Can you work these out from the model? Positions are in its coordinate system, mm. A direction names the side the tool comes from. Coordinates: 2 decimals unless noted, no trailing zeros. Order: outer loops, then holes, each group sorted by start corner. A loop starts at its lowest first (then second) coordinate and runs counter-clockwise, first axis right, second up. Notation, with made-up numbers: (39, 73) -> (44, 73) arc R22 ccw to (44, 96) -> close; hole circle Ø3 at (44, -30). An arc over 180 degrees is marked (long way). Write item = value, one per line.
```python
from build123d import *

# Parameters (mm, degrees)
SKETCH_R          = 1.5
PAD_DEPTH         = 8
SKETCH001_W       = 18.9
SKETCH001_H       = 25.2
POCKET_DEPTH      = 0.8
SKETCH002_W       = 15
SKETCH002_H       = 2.5
SKETCH002_W_2     = 10.4
POCKET001_DEPTH   = 3
SKETCH003_W       = 6
SKETCH003_H       = 30
PAD001_DEPTH      = 9
SKETCH004_W       = 19.2
SKETCH004_H       = 1
POCKET002_DEPTH   = 2
POCKET003_DEPTH   = 3
PAD002_DEPTH      = 3
PAD002_DEPTH_BACK = 3
PAD003_DEPTH      = 1
CHAMFER_SIZE      = 0.95


with BuildPart() as part:
    # Sketch → Pad (new body)
    with BuildSketch(Plane.XY):
        Polygon((-20.1, 15), (11.9, 15), (30, 3.75), (30, -3.75), (11.9, -15), (-20.1, -15), align=None)
        with Locations((-6.25, 0)):
            Circle(SKETCH_R, mode=Mode.SUBTRACT)
    extrude(amount=-PAD_DEPTH)

    # Sketch001 → Pocket (cut)
    with BuildSketch(Plane.XY):
        Rectangle(SKETCH001_W, SKETCH001_H)
    extrude(amount=-POCKET_DEPTH, mode=Mode.SUBTRACT)

    # Sketch002 (on Face33 of Pad003) → Pocket001 (cut)
    with BuildSketch(Plane.XY.offset(-0.8)):
        with Locations((-0.534042, 8.083783)):
            Rectangle(SKETCH002_W, SKETCH002_H)
        with Locations((2.090713, -8.153236)):
            Rectangle(SKETCH002_W_2, SKETCH002_H)
    extrude(amount=-POCKET001_DEPTH, mode=Mode.SUBTRACT)

    # Sketch003 (on Face4 of Pocket001) → Pad001 (join)
    with BuildSketch(Plane.XY):
        with Locations((-17.1, 0)):
            Rectangle(SKETCH003_W, SKETCH003_H)
    extrude(amount=PAD001_DEPTH)

    # Sketch004 (on Face10 of Pad001) → Pocket002 (cut)
    with BuildSketch(Plane.YZ.offset(-14.1)):
        with Locations((0, 5.64)):
            Rectangle(SKETCH004_W, SKETCH004_H)
    extrude(amount=-POCKET002_DEPTH, mode=Mode.SUBTRACT)

    # Sketch005 → Pocket003 (cut)
    with BuildSketch(Plane(origin=(0, 0, -8), x_dir=(1, 0, 0), z_dir=(0, 0, -1))):
        Polygon((-4.633419, 2.8), (-7.866581, 2.8), (-9.483162, 0), (-7.866581, -2.8), (-4.633419, -2.8), (-3.016838, 0), align=None)
    extrude(amount=-POCKET003_DEPTH, mode=Mode.SUBTRACT)

    # Sketch006 → Pad002 (join, two sides)
    with BuildSketch(Plane.XZ) as pad002_sk:
        Polygon((13.9, 0), (20.9, 5.25), (26.9, 5.25), (26.9, 0), align=None)
    extrude(amount=PAD002_DEPTH)
    extrude(pad002_sk.sketch, amount=-PAD002_DEPTH_BACK)

    # Sketch007 (on Face32 of Pad002) → Pad003 (join)
    with BuildSketch(Plane.XY.offset(5.25)):
        with BuildLine():
            ThreePointArc((24, -1.925), (25.925, 0), (24, 1.925))
            Line((24, 1.925), (23, 1.925))
            Line((23, 1.925), (23, -1.925))
            Line((23, -1.925), (24, -1.925))
        make_face()
    extrude(amount=PAD003_DEPTH)

    # Chamfer
    chamfer_edges = [part.edges().sort_by_distance(p)[0] for p in [
        (23, 0, 6.25),
        (23, -1.925, 5.75),
        (23, 1.925, 5.75),
    ]]
    chamfer(chamfer_edges, length=CHAMFER_SIZE)


solid = part.part
```
Item 1: I want a section at A-A, the plane x = -6.25. Please give me the cut outline in (y, z).
A:
outline = (-15, -8) -> (-2.8, -8) -> (-2.8, -5) -> (-1.5, -5) -> (-1.5, -0.8) -> (-12.6, -0.8) -> (-12.6, 0) -> (-15, 0) -> close; (1.5, -5) -> (2.8, -5) -> (2.8, -8) -> (15, -8) -> (15, 0) -> (12.6, 0) -> (12.6, -0.8) -> (9.33, -0.8) -> (9.33, -3.8) -> (6.83, -3.8) -> (6.83, -0.8) -> (1.5, -0.8) -> close
Item 2: If I drill on probe 1 along Y at (x, z) = (-6.25, -2.85); probe 2 along X at (y, z) = (-2.75, -0.75); probe 3 along Z at (x, y) = (5, -2), over which ranges is the centre line in solid material (lowest first)?
A:
probe_1 = -15 to -1.5, 1.5 to 6.83, 9.33 to 15
probe_2 = -20.1 to -9.45, 9.45 to 30
probe_3 = -8 to -0.8
Item 3: I'm going to push flat-ended pins straight in: P1, Ø2, axis at x = -10.5, y = 12, coming from the +Z side; P2, Ø1.8, axis at x = 23, y = 1, coming from the +Z side; P3, Ø4, axis at y = -8.5, z = -4, coming from the +X side. Where does each tip first touch, or does it pass through?
A:
P1 = 0
P2 = 6.2
P3 = 25.58
Item 4: I want a section at D-D, the plane x = 22. Please give me the cut outline in (y, z), plus the area to 3 significant figures.
A:
outline = (-8.72, -8) -> (8.72, -8) -> (8.72, 0) -> (3, 0) -> (3, 5.25) -> (-3, 5.25) -> (-3, 0) -> (-8.72, 0) -> close
area = 171 mm2
Item 5: For faces 5 (the flat face through (26.9, 0, 3)), 6 (the flat face through (-15.1, 9.6, 5.6)), 7 (the flat face through (-8.034, 8, -2)), which set-ups out of +Z, -Z, +X, -X, +Y, -Y let a thin tool reach every point of the face, with its end or its side?
A:
face_5 = +Z, +X, +Y, -Y
face_6 = +X
face_7 = +Z
Item 6: I want a section at B-B, the plane z = -7. Please give me the cut outline in (x, y).
A:
outline = (-20.1, -15) -> (11.9, -15) -> (30, -3.75) -> (30, 3.75) -> (11.9, 15) -> (-20.1, 15) -> close; hole (-9.48, 0) -> (-7.87, -2.8) -> (-4.63, -2.8) -> (-3.02, 0) -> (-4.63, 2.8) -> (-7.87, 2.8) -> close
Item 7: If we mould it in two halves opening along Y, with no side actions, what happens to faces 1 (the flat face through (-3.814, -1.38, -6.521)), 2 (the flat face through (6.966, 8, -2)), 3 (the flat face through (22, -3, 2)), 4 (the flat face through (-8, 15, -3))? For each: pulls with the +Y half, pulls with the -Y half, needs draft (parallel to the pull), parting line crosses it, or undercut.
A:
face_1 = undercut
face_2 = undercut
face_3 = pulls with the -Y half
face_4 = pulls with the +Y half
Item 8: I want a section at C-C, the plane z = 1.5. Please give me the cut outline in (x, y), plus the area to 3 significant figures.
A:
outline = (-20.1, -15) -> (-14.1, -15) -> (-14.1, 15) -> (-20.1, 15) -> close; (15.9, -3) -> (26.9, -3) -> (26.9, 3) -> (15.9, 3) -> close
area = 246 mm2
